Geometry: see drawing. Coordinates: mm, zero at the bounding-box minimum. A direction names the side the tool comes from. Give positions to 0.01 mm unless a question says otherwise; leave off trailing zeros. Order: outer loops, then holes, each group sorted by start corner. A loop starts at its lowest first (then second) coordinate and runs counter-clockwise, first axis right, second up. Notation, with made-up numbers: (80, 52.25) - (90, 52.25) arc R25 cw to (90, 79.25) - close; hole circle Ø10 at (32, 11.25). An arc over 180 degrees is marked (long way). Write item = value, one per line. Start each with the question number.
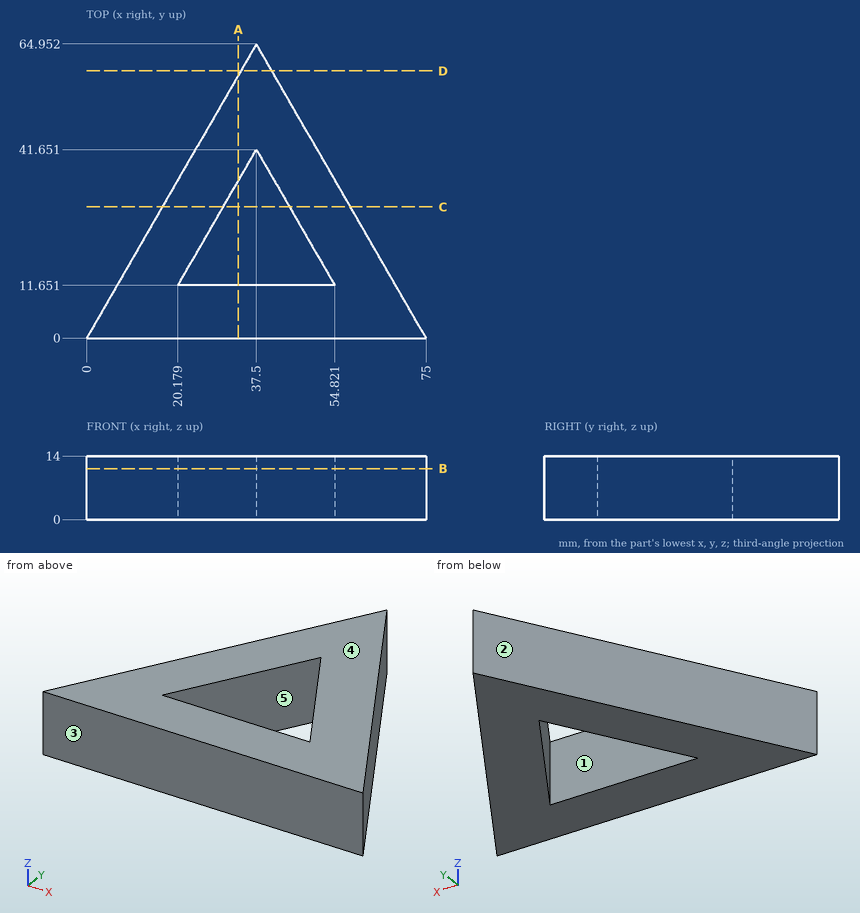
Q1. Section A-A, the plane x = 33.5. Return the cut outline in (y, z), then the cut area to 3 significant figures.
Q2. Section D-D, the plane y = 59. Return the cut outline in (x, z).
Q3. Set-up query: the marked faces 4 and 5. Return all of +Z, -Z, +X, -X, +Y, -Y with unobstructed straight access to the full face (end or side cutting, diameter ignored); none if empty.
Q4. Contact query for flat-ended pins moving along their axis: pin 1 (6 mm diameter, centred on y = 57.5, z = 4, fed in from -X) (1 decimal); pin 2 (5 mm diameter, centred on x = 52, z = 7.5, fed in from +Y) (1 decimal); pin 3 (1 mm diameter, centred on y = 53, z = 1.5, fed in from -X). Output: stop coordinate, or through.
Q5. Pull-direction query (X, two-part tool) for the marked faces 1, 2 and 3; classes: +X half, -X half, draft (parallel to the pull), parting line (faces both ways), or undercut.
Q6. Section B-B, the plane z = 11.25. Return the cut outline in (x, y), then the cut area to 3 significant figures.
Q7. Section C-C, the plane y = 29. Return the cut outline in (x, z), then the cut area to 3 significant figures.
Q8. Material intervals for line 1 along X through (y, z) = (28, 9.5) (1 decimal); line 2 along X through (y, z) = (16, 12.5); line 3 along Y through (x, z) = (15, 3) (1 decimal), sorted ascending. Write a range as from..to.
The answers:
q1.outline = (0, 0) - (11.65, 0) - (11.65, 14) - (0, 14) - close; (34.72, 0) - (58.02, 0) - (58.02, 14) - (34.72, 14) - close
q1.area = 489 mm²
q2.outline = (34.06, 0) - (40.94, 0) - (40.94, 14) - (34.06, 14) - close
q3.face_4 = +Z, +X, -X, +Y, -Y
q3.face_5 = +Z, -Z
q4.pin_1 = 31.5
q4.pin_2 = 44.2
q4.pin_3 = 30.31
q5.face_1 = undercut
q5.face_2 = -X half
q5.face_3 = draft
q6.outline = (0, 0) - (75, 0) - (37.5, 64.95) - close; hole (20.18, 11.65) - (54.82, 11.65) - (37.5, 41.65) - close
q6.area = 1,920 mm²
q7.outline = (16.74, 0) - (30.2, 0) - (30.2, 14) - (16.74, 14) - close; (44.8, 0) - (58.26, 0) - (58.26, 14) - (44.8, 14) - close
q7.area = 377 mm²
q8.line_1 = 16.2..29.6, 45.4..58.8
q8.line_2 = 9.24..22.69, 52.31..65.76
q8.line_3 = 0..26
